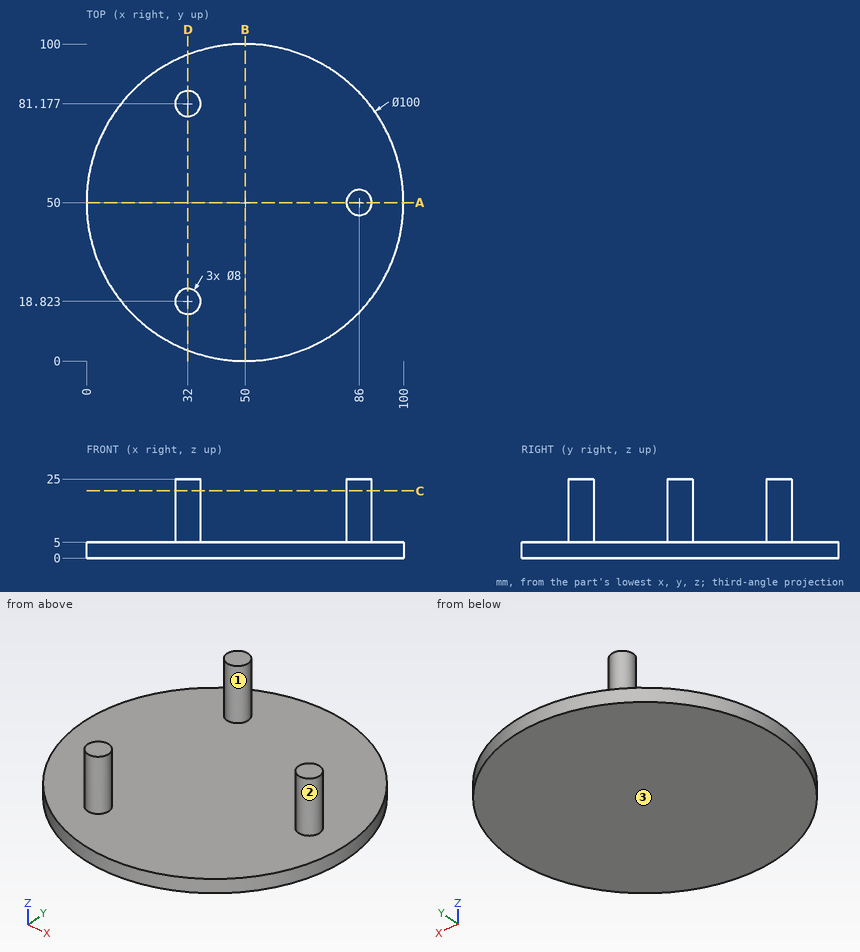
For this review, use the dimensioned drawing (mm, ordinates from the lowest corner) and the shaded views. Round coordinates to 2 decimals unless told otherwise and drop trailing zeros. Write each loop counter-clockwise with the first axis right and the second up, starting at its lowest first coordinate (ties: lowest second). Pieces come first, ordered by that corner, then holes. Notation, with made-up numbers: (-39, -12.75) - (0, -12.75) arc R7 ccw to (0, -4.75) - close; hole circle Ø1 at (-23.75, 14). An arc over 180 degrees is marked (long way). Answer as a JSON object with one key per item and string values.
1. We need section C-C on z = 21.25. Give the boundary of the cut face in (x, y), then the cut area to 3 significant figures.
Response values:
{"outline": "circle Ø8 at (32, 18.82); circle Ø8 at (32, 81.18); circle Ø8 at (86, 50)", "area": "151 mm2"}
2. We need section D-D on x = 32. Give the boundary of the cut face in (y, z).
Response values:
{"outline": "(3.35, 0) - (96.65, 0) - (96.65, 5) - (85.18, 5) - (85.18, 25) - (77.18, 25) - (77.18, 5) - (22.82, 5) - (22.82, 25) - (14.82, 25) - (14.82, 5) - (3.35, 5) - close"}
3. We need section A-A on y = 50. Give the boundary of the cut face in (x, z), then the cut area to 3 significant figures.
Response values:
{"outline": "(0, 0) - (100, 0) - (100, 5) - (90, 5) - (90, 25) - (82, 25) - (82, 5) - (0, 5) - close", "area": "660 mm2"}
4. We need section B-B on x = 50. Give the boundary of the cut face in (y, z).
Response values:
{"outline": "(0, 0) - (100, 0) - (100, 5) - (0, 5) - close"}
5. To check wall thickness, follow line 1 along Y through (x, z) = (35.5, 10); line 2 along Z through (x, y) = (18, 43.5); line 3 along X through (y, z) = (53.5, 15.5). State the ranges of each line that lie inside material, in increasing order.
Response values:
{"line 1": "y = 16.89 to 20.76, 79.24 to 83.11", "line 2": "z = 0 to 5", "line 3": "x = 84.06 to 87.94"}
6. For pin 1 Ø10 at (y, z) = (71, 3) entering from -X; pin 2 Ø12 at (y, z) = (54.5, 14) entering from +X; pin 3 Ø5 at (x, y) = (48, 57) entering from +Z, all flat-tipped, find the tip position at first contact; note any pin that passes through.
Response values:
{"pin 1": "stops at x = 2.63", "pin 2": "stops at x = 90", "pin 3": "stops at z = 5"}
7. Draft analysis for pull direction Y (two halves, no side actions). For the marked faces 1, 2 and 3, state which applies: +Y half, -Y half, draft (parallel to the pull), parting line (faces both ways), or undercut.
Response values:
{"face 1": "undercut", "face 2": "parting line", "face 3": "draft"}
